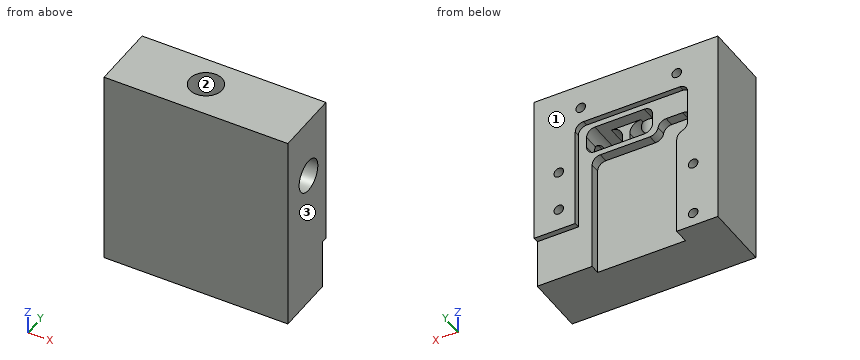
```python
from build123d import *

# Parameters (mm, degrees)
SKETCH1_W                = 67
SKETCH1_H                = 73
BOSS_EXTRUDE1_DEPTH      = 15
BOSS_EXTRUDE2_DEPTH      = 3.5
SKETCH6_W                = 24
SKETCH6_H                = 10
CUT_EXTRUDE2_DEPTH       = 16
SKETCH11_W               = 67
SKETCH11_H               = 73
BOSS_EXTRUDE4_DEPTH      = 3.5
SKETCH13_W               = 15
SKETCH13_H               = 40
BOSS_EXTRUDE6_DEPTH      = 5.5
SKETCH14_R               = 1.75
CUT_EXTRUDE7_DEPTH       = 10
BOSS_EXTRUDE7_DEPTH      = 5.5
FILLET5_R                = 3
SKETCH20_W               = 15
SKETCH20_H               = 18
BOSS_EXTRUDE8_DEPTH      = 3.5
FILLET10_R               = 3
FILLET11_R               = 3
FILLET12_R               = 3
FILLET13_R               = 3
SKETCH21_W               = 2.649172372
SKETCH21_H               = 10
BOSS_EXTRUDE9_DEPTH      = 12
FILLET15_R               = 4
SKETCH19_R               = 1.75
CUT_EXTRUDE11_DEPTH      = 10
SKETCH23_R               = 4
CUT_EXTRUDE12_DEPTH      = 2
CUT_EXTRUDE12_DEPTH_BACK = 91.278735196
SKETCH24_R               = 5.9
CUT_EXTRUDE13_DEPTH      = 10
SKETCH25_R               = 4
CUT_EXTRUDE14_DEPTH      = 2
CUT_EXTRUDE14_DEPTH_BACK = 90.695317764
SKETCH26_R               = 5.9
CUT_EXTRUDE15_DEPTH      = 10


with BuildPart() as part:
    # Sketch1 → Boss-Extrude1 (new body)
    with BuildSketch(Plane(origin=(0, 0, 0), x_dir=(1, 0, 0), z_dir=(0, 1, 0))):
        with Locations((33.5, 36.5)):
            Rectangle(SKETCH1_W, SKETCH1_H)
    extrude(amount=BOSS_EXTRUDE1_DEPTH)

    # Sketch5 → Boss-Extrude2 (add)
    with BuildSketch(Plane(origin=(0, 15, 0), x_dir=(1, 0, 0), z_dir=(0, 1, 0))):
        with BuildLine():
            Line((18.5, 15), (11, 15))
            Line((11, 15), (11, 24))
            Line((11, 24), (14.788897449, 24))
            Line((14.788897449, 24), (20, 24))
            ThreePointArc((20, 24), (22.121320344, 24.878679656), (23, 27))
            Line((23, 27), (23, 29))
            Line((23, 29), (47, 29))
            Line((47, 29), (47, 73))
            Line((47, 73), (52, 73))
            Line((52, 73), (52, 15))
            Line((52, 15), (32, 15))
            Line((32, 15), (18.5, 15))
        make_face()
    extrude(amount=BOSS_EXTRUDE2_DEPTH)

    # Sketch6 → Cut-Extrude2 (cut)
    with BuildSketch(Plane(origin=(0, 18.5, 0), x_dir=(1, 0, 0), z_dir=(0, 1, 0))):
        with Locations((37, 22)):
            Rectangle(SKETCH6_W, SKETCH6_H)
    extrude(amount=-CUT_EXTRUDE2_DEPTH, mode=Mode.SUBTRACT)

    # Sketch11 → Boss-Extrude4 (add)
    with BuildSketch(Plane.XZ):
        with Locations((33.5, -36.5)):
            Rectangle(SKETCH11_W, SKETCH11_H)
    extrude(amount=BOSS_EXTRUDE4_DEPTH)

    # Sketch13 → Boss-Extrude6 (add)
    with BuildSketch(Plane(origin=(0, 15, 0), x_dir=(1, 0, 0), z_dir=(0, 1, 0))):
        with Locations((59.5, 35)):
            Rectangle(SKETCH13_W, SKETCH13_H)
    extrude(amount=BOSS_EXTRUDE6_DEPTH)

    # Sketch14 → Cut-Extrude7 (cut)
    with BuildSketch(Plane(origin=(0, 20.5, 0), x_dir=(1, 0, 0), z_dir=(0, 1, 0))):
        with Locations(Location((58, 47, 0), (0, 0, 270))):
            Circle(SKETCH14_R)
        with Locations(Location((58, 32, 0), (0, 0, 270))):
            Circle(SKETCH14_R)
    extrude(amount=-CUT_EXTRUDE7_DEPTH, mode=Mode.SUBTRACT)

    # Sketch18 → Boss-Extrude7 (add)
    with BuildSketch(Plane(origin=(0, 15, 0), x_dir=(1, 0, 0), z_dir=(0, 1, 0))):
        with BuildLine():
            Line((15, 33.237791503), (15, 73))
            Line((15, 73), (0, 73))
            Line((0, 73), (0, 15))
            Line((0, 15), (0, 0))
            Line((0, 0), (67, 0))
            Line((67, 0), (67, 15))
            Line((67, 15), (15, 15))
            Line((15, 15), (13.782507359, 15))
            ThreePointArc((13.782507359, 15), (11.803129735, 15.9491273), (11, 17.992105772))
            Line((11, 17.992105772), (11, 30.237791503))
            ThreePointArc((11, 30.237791503), (11.878679656, 32.359111846), (14, 33.237791503))
            Line((14, 33.237791503), (15, 33.237791503))
        make_face()
    extrude(amount=BOSS_EXTRUDE7_DEPTH)

    # Fillet5
    fillet5_edges = [part.edges().sort_by_distance(p)[0] for p in [
        (52, 19.5, -15),
    ]]
    fillet(fillet5_edges, radius=FILLET5_R)

    # Sketch20 → Boss-Extrude8 (add)
    with BuildSketch(Plane(origin=(0, 15, 0), x_dir=(1, 0, 0), z_dir=(0, 1, 0))):
        with Locations((59.5, 64)):
            Rectangle(SKETCH20_W, SKETCH20_H)
    extrude(amount=BOSS_EXTRUDE8_DEPTH)

    # Fillet10
    fillet10_edges = [part.edges().sort_by_distance(p)[0] for p in [
        (47, 16.75, -29),
    ]]
    fillet(fillet10_edges, radius=FILLET10_R)

    # Fillet11
    fillet11_edges = [part.edges().sort_by_distance(p)[0] for p in [
        (23, 16.75, -29),
        (11, 16.75, -24),
    ]]
    fillet(fillet11_edges, radius=FILLET11_R)

    # Fillet12
    fillet12_edges = [part.edges().sort_by_distance(p)[0] for p in [
        (15, 17.75, -33.237791503),
    ]]
    fillet(fillet12_edges, radius=FILLET12_R)

    # Fillet13
    fillet13_edges = [part.edges().sort_by_distance(p)[0] for p in [
        (25, 10.5, -17),
        (25, 10.5, -27),
        (49, 10.5, -27),
        (49, 10.5, -17),
    ]]
    fillet(fillet13_edges, radius=FILLET13_R)

    # Sketch21 → Boss-Extrude9 (add)
    with BuildSketch(Plane(origin=(0, 2.5, 0), x_dir=(1, 0, 0), z_dir=(0, 1, 0))):
        with Locations((36.905299385, 22)):
            Rectangle(SKETCH21_W, SKETCH21_H)
    extrude(amount=BOSS_EXTRUDE9_DEPTH)

    # Fillet15
    fillet15_edges = [part.edges().sort_by_distance(p)[0] for p in [
        (35.580713199, 8.5, -27),
        (35.580713199, 8.5, -17),
        (38.229885571, 8.5, -17),
        (38.229885571, 8.5, -27),
    ]]
    fillet(fillet15_edges, radius=FILLET15_R)

    # Sketch19 → Cut-Extrude11 (cut)
    with BuildSketch(Plane(origin=(0, 20.5, 0), x_dir=(1, 0, 0), z_dir=(0, 1, 0))):
        with Locations(Location((9, 48, 0), (0, 0, 270))):
            Circle(SKETCH19_R)
        with Locations(Location((9, 68, 0), (0, 0, 270))):
            Circle(SKETCH19_R)
        with Locations(Location((15, 9, 0), (0, 0, 270))):
            Circle(SKETCH19_R)
        with Locations(Location((50, 9, 0), (0, 0, 270))):
            Circle(SKETCH19_R)
    extrude(amount=-CUT_EXTRUDE11_DEPTH, mode=Mode.SUBTRACT)

    # Sketch23 → Cut-Extrude12 (cut, two sides)
    with BuildSketch(Plane.ZY.offset(-49)) as cut_extrude12_sk:
        with Locations(Location((-22, 9.5, 0), (0, 0, 240))):
            Circle(SKETCH23_R)
    extrude(amount=CUT_EXTRUDE12_DEPTH, mode=Mode.SUBTRACT)
    extrude(cut_extrude12_sk.sketch, amount=-CUT_EXTRUDE12_DEPTH_BACK, mode=Mode.SUBTRACT)

    # Sketch24 → Cut-Extrude13 (cut)
    with BuildSketch(Plane(origin=(67, 0, 0), x_dir=(0, 0, -1), z_dir=(1, 0, 0))):
        with Locations((22, 9.5)):
            Circle(SKETCH24_R)
    extrude(amount=-CUT_EXTRUDE13_DEPTH, mode=Mode.SUBTRACT)

    # Sketch25 → Cut-Extrude14 (cut, two sides)
    with BuildSketch(Plane(origin=(0, 0, -17), x_dir=(-1, 0, 0), z_dir=(0, 0, -1))) as cut_extrude14_sk:
        with Locations(Location((-29.628343357, 9.5, 0), (0, 0, 240.784718546))):
            Circle(SKETCH25_R)
    extrude(amount=CUT_EXTRUDE14_DEPTH, mode=Mode.SUBTRACT)
    extrude(cut_extrude14_sk.sketch, amount=-CUT_EXTRUDE14_DEPTH_BACK, mode=Mode.SUBTRACT)

    # Sketch26 → Cut-Extrude15 (cut)
    with BuildSketch(Plane.XY):
        with Locations((29.628343357, 9.5)):
            Circle(SKETCH26_R)
    extrude(amount=-CUT_EXTRUDE15_DEPTH, mode=Mode.SUBTRACT)


solid = part.part
```
Build history of the part. All positions in model axes, mm. Face numbers are marked on the shaded views. Round coordinates to 2 decimals unless told otherwise and drop trailing zeros. Order: outer loops, then holes, each group sorted by start corner. A loop starts at its lowest first (then second) coordinate and runs counter-clockwise, first axis right, second up. Notation, with made-up numbers: (43, -16.75) - (72, -16.75) arc R12 ccw to (72, -10.75) - close; hole circle Ø1 at (51, 72.25). An arc over 180 degrees is marked (long way). Use a Markdown table: item, result.
1) Flat gauge pins, fed straight in: pin 1 Ø11 at (x, z) = (44, -21) entering from +Y; pin 2 Ø1 at (y, z) = (8.5, -22.5) entering from +X; pin 3 Ø5 at (x, z) = (36, -23) entering from +Y. Where does each tip first touch, or does it go through?
Recorded:
| item | result |
|---|---|
| pin 1 | stops at y = 18.5 |
| pin 2 | stops at x = 38.23 |
| pin 3 | stops at y = 14.5 |
2) Pull direction Y, two halves, no side cores. Call the marked faces 1, 2 and 3: pulls with the +Y half, pulls with the -Y half, needs draft (parallel to the pull), parting line crosses it, or undercut.
Recorded:
| item | result |
|---|---|
| face 1 | pulls with the +Y half |
| face 2 | undercut |
| face 3 | needs draft |
3) Wall check: L1, parallel to X at y = 17.5, z = -9; L2, parallel to X at y = 9.5, z = -13.75; L3, parallel to X at y = 15.25, z = -32. Give the ranges that are in metal, low to high.
Recorded:
| item | result |
|---|---|
| L1 | x = 0 to 13.25, 16.75 to 48.25, 51.75 to 67 |
| L2 | x = 0 to 25.63, 33.63 to 67 |
| L3 | x = 0 to 11.57, 47 to 56.25, 59.75 to 67 |
4) Saw through at D-D on z = -9. Write the cut outline in (x, y), and give its area (3 significant figures).
Recorded:
| item | result |
|---|---|
| outline | (0, -3.5) - (67, -3.5) - (67, 20.5) - (51.75, 20.5) - (51.75, 10.5) - (48.25, 10.5) - (48.25, 20.5) - (16.75, 20.5) - (16.75, 10.5) - (13.25, 10.5) - (13.25, 20.5) - (0, 20.5) - close; hole circle Ø11.8 at (29.63, 9.5) |
| area | 1,430 mm² |
5) Saw through at C-C on z = -37. Write the cut outline in (x, y).
Recorded:
| item | result |
|---|---|
| outline | (0, -3.5) - (67, -3.5) - (67, 20.5) - (52, 20.5) - (52, 18.5) - (47, 18.5) - (47, 15) - (15, 15) - (15, 20.5) - (0, 20.5) - close |
6) Saw through at B-B on z = -22. Write the cut outline in (x, y), and give its area (3 significant figures).
Recorded:
| item | result |
|---|---|
| outline | (0, -3.5) - (67, -3.5) - (67, 3.6) - (57, 3.6) - (57, 5.5) - (49, 5.5) - (49, 2.5) - (38.23, 2.5) - (38.23, 14.5) - (35.58, 14.5) - (35.58, 2.5) - (25, 2.5) - (25, 18.5) - (11, 18.5) - (11, 20.5) - (0, 20.5) - close; (49, 13.5) - (57, 13.5) - (57, 15.4) - (67, 15.4) - (67, 20.5) - (52, 20.5) - (52, 18.5) - (49, 18.5) - close |
| area | 992 mm² |
7) Saw through at A-A on x = 63. Write the cut outline in (y, z), and give its area (3 significant figures).
Recorded:
| item | result |
|---|---|
| outline | (-3.5, -73) - (18.5, -73) - (18.5, -55) - (20.5, -55) - (20.5, 0) - (-3.5, 0) - close; hole circle Ø11.8 at (9.5, -22) |
| area | 1,610 mm² |
